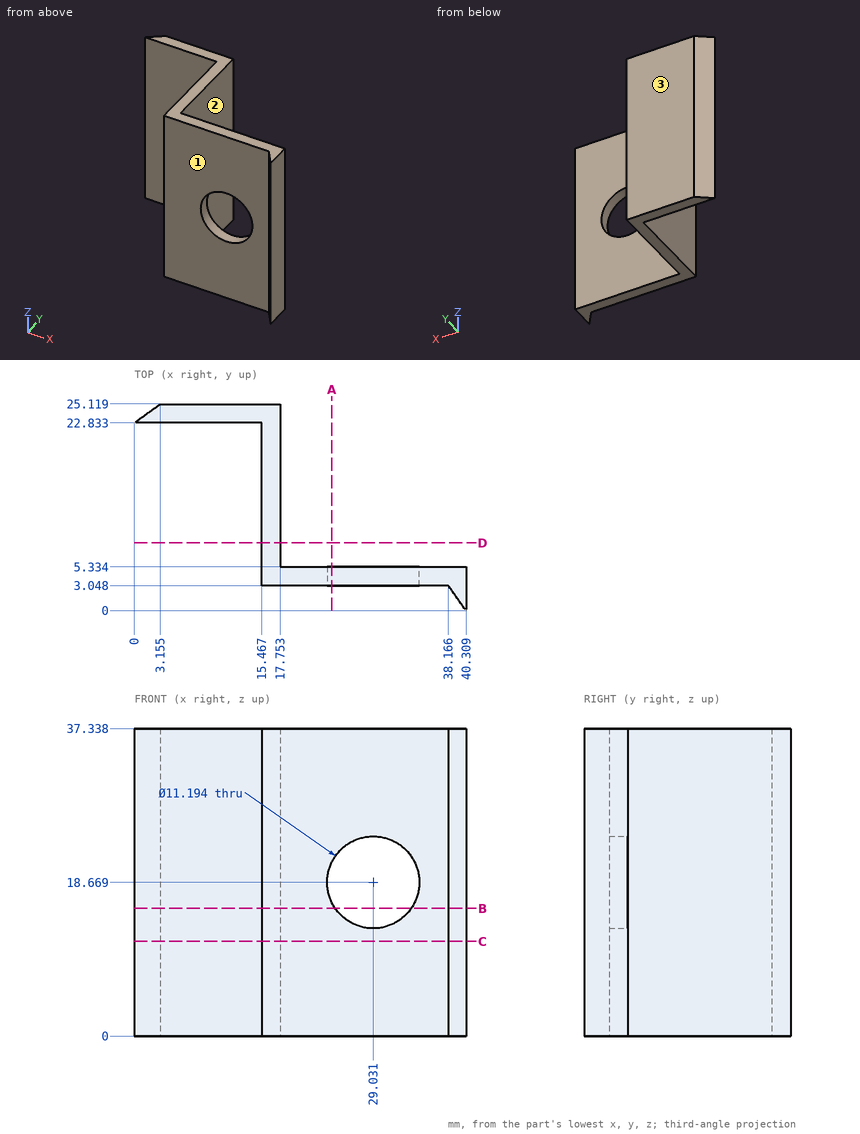
Job drawing, mm, ordinate dimensions from the low corner. One solid piece. A direction names the side the tool comes from. Coordinates: 2 decimals unless noted, no trailing zeros. Write each loop counter-clockwise with the first axis right and the second up, starting at its lowest first coordinate (ties: lowest second). Pieces come first, ordered by that corner, then holes.
Item 1: Slice it at C-C (z = 11.5). Write the cut outline in (x, y) (1 decimal), and give its area (3 significant figures).
Item 2: Pin check, flat tips, straight feed: pin 1 (10 mm diameter, centred on y = 14.5, z = 17.5, fed in from +X); pin 2 (2 mm diameter, centred on x = 22.5, z = 17, fed in from +Y); pin 3 (10 mm diameter, centred on x = 8, y = 8.5, fed in from +Z); pin 4 (13 mm diameter, centred on x = 29.03, z = 18.67, fed in from -Y). Stop position of each tip, or through.
Item 3: Slice it at B-B (z = 15.5). Write the cut outline in (x, y) (1 decimal).
Item 4: Slice it at D-D (y = 8.25). Write the cut outline in (x, z).
Item 5: Probe line 1 (X direction, y = 4.25, z = 7.5); line 2 (X direction, y = 22, z = 26); line 3 (Y direction, x = 15, z = 25). List the from-to ranges inside material, lowest first.
Item 6: Slice it at A-A (x = 24). Write the cut outline in (y, z).
Item 7: Which spindle directions (+Z, -Z, +X, -X, +Y, -Y) get a long thin tool onto all of the face, cutting with end or side? Do the marked faces 1, 2 and 3. Say none if no direction does.
Results found:
1. outline: (0, 22.8) - (15.5, 22.8) - (15.5, 3) - (38.2, 3) - (40.3, 0) - (40.3, 5.3) - (17.8, 5.3) - (17.8, 25.1) - (3.2, 25.1) - close
1. area: 137 mm2
2. pin 1: stops at x = 17.75
2. pin 2: stops at y = 5.33
2. pin 3: passes through
2. pin 4: stops at y = 3.05
3. outline: (0, 22.8) - (15.5, 22.8) - (15.5, 3) - (24.4, 3) - (24.4, 5.3) - (17.8, 5.3) - (17.8, 25.1) - (3.2, 25.1) - close; (33.6, 3) - (38.2, 3) - (40.3, 0) - (40.3, 5.3) - (33.6, 5.3) - close
4. outline: (15.47, 0) - (17.75, 0) - (17.75, 37.34) - (15.47, 37.34) - close
5. line 1: x = 15.47 to 40.31
5. line 2: x = 15.47 to 17.75
5. line 3: y = 22.83 to 25.12
6. outline: (3.05, 0) - (5.33, 0) - (5.33, 16.22) - (3.05, 16.22) - close; (3.05, 21.12) - (5.33, 21.12) - (5.33, 37.34) - (3.05, 37.34) - close
7. face 1: +Z, -Z, -X, -Y
7. face 2: +Z, -Z, +X, +Y
7. face 3: +Z, -Z, +X, -X, +Y
